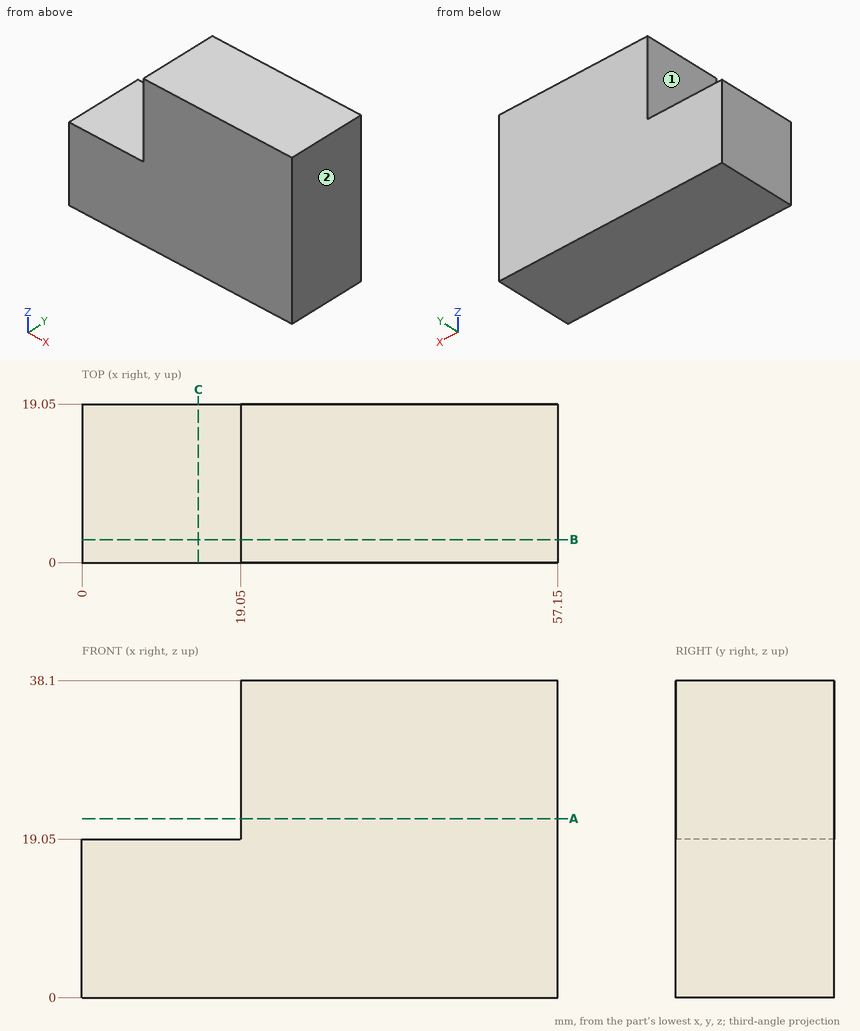
Here's the drawing with two shaded views (mm, measured from the low corner). I have some questions. A direction names the side the tool comes from. Coordinates: 2 decimals unless noted, no trailing zeros. Order: outer loops, then holes, each group sorted by start corner. A loop starts at its lowest first (then second) coordinate and runs counter-clockwise, first axis right, second up. Notation, with made-up numbers: (-39, 43) -> (0, 43) arc R31 cw to (0, 71) -> close; hole circle Ø11 at (34, 20). An arc over 180 degrees is marked (long way). One line per question, with ' | ' between items.
Q1. If I drill on L1, parallel to X at y = 1.75, z = 33; L2, parallel to Z at x = 10, y = 14, over which ranges is the centre line in solid material (lowest first)?
Return value:
L1: 19.05 to 57.15 | L2: 0 to 19.05
Q2. I'm going to push a flat-ended pin straight in: P1, Ø9.5, axis at x = 6, y = 6, coming from the +Z side. Where does the tip first touch, or does it pass through?
Return value:
P1: z = 19.05
Q3. Imagine slicing it at B-B on y = 2.75. Please give me the cut outline in (x, z), and give its area (3 significant figures).
Return value:
outline: (0, 0) -> (57.15, 0) -> (57.15, 38.1) -> (19.05, 38.1) -> (19.05, 19.05) -> (0, 19.05) -> close | area: 1,810 mm²
Q4. Imagine slicing it at A-A on z = 21.5. Please give me the cut outline in (x, y).
Return value:
outline: (19.05, 0) -> (57.15, 0) -> (57.15, 19.05) -> (19.05, 19.05) -> close
Q5. On a 3-axis mill with a long thin cutter (end or side, diameter ignored), from which of +Z, -Z, +X, -X, +Y, -Y can I reach the whole of each face in a straight line? I mean the marked faces 1 and 2. Say none if no direction works.
Return value:
face 1: +Z, -X, +Y, -Y | face 2: +Z, -Z, +X, +Y, -Y
Q6. Imagine slicing it at C-C on x = 14. Please give me the cut outline in (y, z).
Return value:
outline: (0, 0) -> (19.05, 0) -> (19.05, 19.05) -> (0, 19.05) -> close
